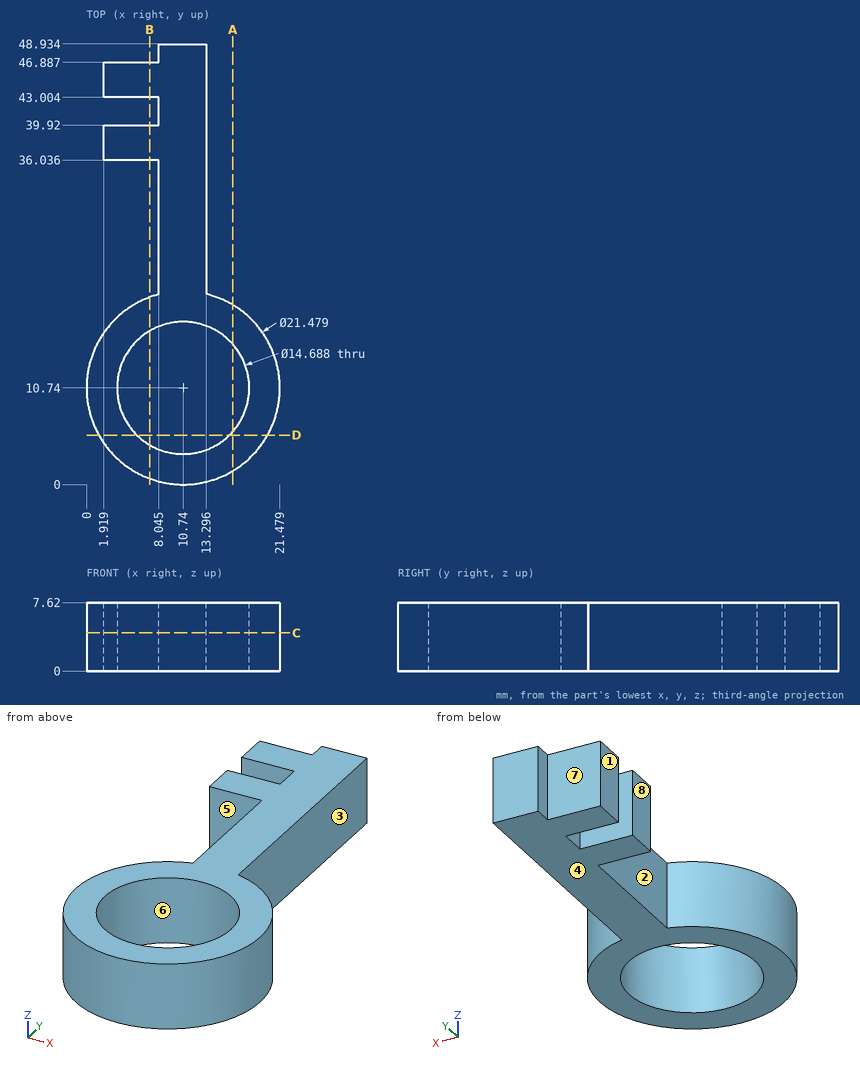
The figure shows three views and two pictorial views of one solid part (mm, origin at its lowest corner). Answer the questions. A direction names the side the tool comes from. Give positions to 0.01 mm unless a question says otherwise; leave off trailing zeros. Loops run counter-clockwise (first coordinate to the right, second up) from the corner with the lowest first, then second, coordinate; pieces in that order, holes last. Notation, with made-up numbers: (76.5, 25) -> (87.5, 25) arc R20 cw to (87.5, 58) -> close; hole circle Ø8 at (30, 4.25). An arc over 180 degrees is marked (long way). Use CSV: the item, a comma, the result in double quotes.
1. The part is cut by section A-A (x = 16.25). Write down the section's boundary in (y, z) (1 decimal), then the cut area to 3 significant figures.
Found:
outline,"(1.5, 0) -> (5.9, 0) -> (5.9, 7.6) -> (1.5, 7.6) -> close; (15.6, 0) -> (20, 0) -> (20, 7.6) -> (15.6, 7.6) -> close"
area,"66.5 mm^2"
2. The part is cut by section D-D (y = 5.5). Write down the section's boundary in (x, z) (1 decimal).
Found:
outline,"(1.4, 0) -> (5.6, 0) -> (5.6, 7.6) -> (1.4, 7.6) -> close; (15.9, 0) -> (20.1, 0) -> (20.1, 7.6) -> (15.9, 7.6) -> close"
3. The part is cut by section B-B (x = 7). Write down the section's boundary in (y, z) (1 decimal).
Found:
outline,"(0.7, 0) -> (4.4, 0) -> (4.4, 7.6) -> (0.7, 7.6) -> close; (17.1, 0) -> (20.8, 0) -> (20.8, 7.6) -> (17.1, 7.6) -> close; (36, 0) -> (39.9, 0) -> (39.9, 7.6) -> (36, 7.6) -> close; (43, 0) -> (46.9, 0) -> (46.9, 7.6) -> (43, 7.6) -> close"
4. Straight lines are drawn through the part: line 1 (Y direction, x = 8, z = 6.75) (1 decimal); line 2 (Y direction, x = 4.5, z = 5.25) (1 decimal); line 3 (X direction, y = 10.5, z = 2.5). For each, find the intervals that lie inside material, in ascending order.
Found:
line 1,"0.4 to 3.9, 17.6 to 21.1, 36 to 39.9, 43 to 46.9"
line 2,"2 to 6.9, 14.6 to 19.5, 36 to 39.9, 43 to 46.9"
line 3,"0 to 3.4, 18.08 to 21.48"
5. The part is cut by section C-C (z = 4.25). Write down the section's boundary in (x, y) (1 decimal).
Found:
outline,"(1.9, 36) -> (8, 36) -> (8, 21.1) arc R10.7 ccw (long way) to (13.3, 21.2) -> (13.3, 48.9) -> (8, 48.9) -> (8, 46.9) -> (1.9, 46.9) -> (1.9, 43) -> (8, 43) -> (8, 39.9) -> (1.9, 39.9) -> close; hole circle Ø14.7 at (10.7, 10.7)"
6. Flat-ended cylindrical pins translate along their axes: pin 1 Ø1.5 at (y, z) = (42, 2) entering from -X (1 decimal); pin 2 Ø3 at (x, z) = (4, 2) entering from -Y (1 decimal); pin 3 Ø1 at (x, z) = (7.5, 3.5) entering from -Y (1 decimal); pin 4 Ø8 at (x, y) = (9, 8.5) entering from +Z. Find the tip coordinate at first contact, or state that the pin passes through.
Found:
pin 1,"x = 8"
pin 2,"y = 1.4"
pin 3,"y = 0.4"
pin 4,"through"
7. A tool of negligible diameter and unlimited length cuts with its end or side. For the marked faces 1, 2, 3 and 4, from which of +Z, -Z, +X, -X, +Y, -Y can it reach the whole face along a straight path? Write none if from no direction.
Found:
face 1,"+Z, -Z, -X, +Y"
face 2,"+Z, -Z, -X"
face 3,"+Z, -Z, +X, +Y"
face 4,"-Z, +X, -X, +Y, -Y"
8. The mould has two halves that part along Y. Classify the marked faces 5, 6, 7 and 8: +Y half, -Y half, draft (parallel to the pull), parting line (faces both ways), or undercut.
Found:
face 5,"undercut"
face 6,"undercut"
face 7,"+Y half"
face 8,"draft"
